Can you work these out from the model? Positions are in its coordinate system, mm. Coordinates: 2 decimals unless noted, no trailing zeros. Order: outer loops, then holes, each group sorted by start corner. A loop starts at its lowest first (then second) coordinate and runs counter-clockwise, first axis right, second up. Notation, with made-up numbers: (-37, 59) -> (-32, 59) arc R20 cw to (-32, 79) -> close; hole circle Ø6 at (-13.75, 86.5). An arc over 180 degrees is marked (long way). Answer as CSV lines item,"result".
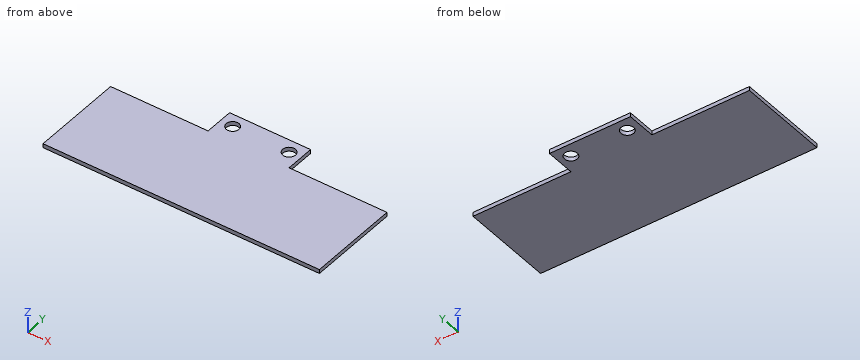
Autodesk Inventor part; units mm, degrees
ref_plane "YZ Plane" through (0, 0, 0) normal (1, 0, 0) x (0, 1, 0)
ref_plane "XZ Plane" through (0, 0, 0) normal (0, 1, 0) x (-1, 0, 0)
ref_plane "XY Plane" through (0, 0, 0) normal (0, 0, 1) x (1, 0, 0)
ref_plane "Work Plane1" through (0, 0, 0) normal (0, 0, 1) x (1, 0, 0)
sketch "Sketch1" plane through (0, 0, 0) normal (0, 0, 1) x (1, 0, 0)
  circle A0 centre (6.766, 15.49) radius 1.5875
  circle A1 centre (-7.234, 15.49) radius 1.5875
  line L0 (-34.544, 11.43) -> (-34.544, -11.43)
  line L1 (-34.544, -11.43) -> (34.036, -11.43)
  line L2 (34.036, -11.43) -> (34.036, 11.43)
  line L3 (-10.3543, 11.43) -> (-10.3543, 18.7046)
  line L4 (-10.3543, 18.7046) -> (9.7417, 18.7046)
  line L5 (9.7417, 18.7046) -> (9.7417, 11.43)
  line L6 (34.036, 11.43) -> (9.7417, 11.43)
  line L7 (-10.3543, 11.43) -> (-34.544, 11.43)
  point P0 (0, 0)
  dimension "d0" = 68.58
  dimension "d1" = 22.86
  dimension "d2" = 27.31
  dimension "d3" = 14
  dimension "d4" = 3.175
  dimension "d5" = 3.175
  dimension "d10" = 26.92
extrude "Extrusion1" add sketch "Sketch1" along normal blind 1
properties part number "Syringe PCB"
Q1. If I drill on line 1 (Y direction, x = 7, z = 0.95); line 2 (X direction, y = 13, z = 0.8); line 3 (Y direction, x = 17, z = 0.6), over which ranges is the centre line in solid material (lowest first)?
Solution:
line 1,"-11.43 to 13.92, 17.06 to 18.7"
line 2,"-10.35 to 9.74"
line 3,"-11.43 to 11.43"
Q2. For P1, Ø0.5, axis at x = -17, z = 0.5, coming from the +Y side, with a flat end and sliding along its axis, tell me the tip position at first contact or that it passes through.
Solution:
P1,"y = 11.43"
Q3. Imagine slicing it at B-B (z = 0.85). List the corners of the cut face in (x, y) for me (1 decimal).
Solution:
outline,"(-34.5, -11.4) -> (34, -11.4) -> (34, 11.4) -> (9.7, 11.4) -> (9.7, 18.7) -> (-10.4, 18.7) -> (-10.4, 11.4) -> (-34.5, 11.4) -> close; hole circle Ø3.2 at (-7.2, 15.5); hole circle Ø3.2 at (6.8, 15.5)"
Q4. Imagine slicing it at C-C (x = -15.5). List the corners of the cut face in (y, z) for me, and give its area (3 significant figures).
Solution:
outline,"(-11.43, 0) -> (11.43, 0) -> (11.43, 1) -> (-11.43, 1) -> close"
area,"22.9 mm2"
Q5. Imagine slicing it at A-A (y = 15.49). List the corners of the cut face in (x, z) for me, and give its area (3 significant figures).
Solution:
outline,"(-10.35, 0) -> (-8.82, 0) -> (-8.82, 1) -> (-10.35, 1) -> close; (-5.65, 0) -> (5.18, 0) -> (5.18, 1) -> (-5.65, 1) -> close; (8.35, 0) -> (9.74, 0) -> (9.74, 1) -> (8.35, 1) -> close"
area,"13.7 mm2"
